Check sheet for the modelled part. Datum: model origin and axes. Units: mm. Coordinates: 2 decimals unless noted, no trailing zeros. Write each loop counter-clockwise with the first axis right and the second up, starting at its lowest first coordinate (ties: lowest second). Pieces come first, ordered by that corner, then holes. Notation, with made-up numbers: (-7, 56.5) - (49, 56.5) arc R23 cw to (49, 81.5) - close; hole circle Ø11 at (69.25, 73.5). An arc over 180 degrees is marked (long way). Use one line per item in the form item = value. Start each with the question number.
1. Scan lines: line 1 along X through (y, z) = (2.45, -15.5); line 2 along Z through (x, y) = (0, 0.75); line 3 along X through (y, z) = (1.8, -12). Record each from-to range of solid material in increasing order.
2. Cross-section at A-A on z = 0. Record the boundary of the cut face in (x, y), then the cut area to 3 significant figures.
3. Cross-section at B-B on x = 0. Record the boundary of the cut face in (y, z), then the cut area to 3 significant figures.
4. Go/stop test with a flat-tipped pin: pin 1 Ø10 at (x, z) = (-37.5, -12) entering from +Y. Record where the tip stops, or that it passes through.
5. Cross-section at C-C on y = 1.7. Give the number of separate pieces and of enclosed holes in the cut face, then the cut area to 3 significant figures.
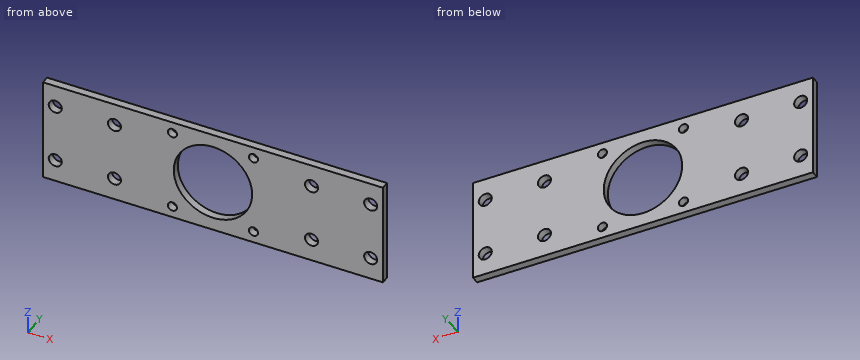
```python
from build123d import *

# Parameters (mm, degrees)
SKETCH1_W                  = 130
SKETCH1_H                  = 40
BOSS_EXTRUDE1_DEPTH        = 3
SKETCH2_R                  = 15
CUT_EXTRUDE1_DEPTH         = 69.0734897
F_5_0_5_DIAMETER_HOLE1_D   = 5
F_3_5_3_5_DIAMETER_HOLE1_D = 3.5


with BuildPart() as part:
    # Sketch1 → Boss-Extrude1 (new body)
    with BuildSketch(Plane(origin=(0, 0, 0), x_dir=(1, 0, 0), z_dir=(0, 1, 0))):
        Rectangle(SKETCH1_W, SKETCH1_H)
    extrude(amount=BOSS_EXTRUDE1_DEPTH)

    # Sketch2 → Cut-Extrude1 (cut, through all)
    with BuildSketch(Plane(origin=(0, 0, 0), x_dir=(1, 0, 0), z_dir=(0, 1, 0))):
        with Locations(Location((0, 0, 0), (0, 0, 270))):
            Circle(SKETCH2_R)
    extrude(amount=CUT_EXTRUDE1_DEPTH, mode=Mode.SUBTRACT)

    # Ø5.0 (5) Diameter Hole1 (through all)
    with Locations(Plane(origin=(0, 0, 0), x_dir=(-1, 0, 0), z_dir=(0, -1, 0))):
        with Locations((60.313708499, 11.313708499), (60.313708499, -11.313708499), (37.686291501, -11.313708499), (37.686291501, 11.313708499)):
            f_5_0_5_diameter_hole1 = Hole(F_5_0_5_DIAMETER_HOLE1_D / 2)

    # Mirror1: Ø5.0 (5) Diameter Hole1 across plane
    add(f_5_0_5_diameter_hole1.mirror(Plane(origin=(0, 0, 0), x_dir=(0, 0, 1), z_dir=(1, 0, 0))), mode=Mode.SUBTRACT)

    # Ø3.5 (3.5) Diameter Hole1 (through all)
    with Locations(Plane(origin=(0, 0, 0), x_dir=(-1, 0, 0), z_dir=(0, -1, 0))):
        with Locations((0, 0), (-15.5, 15.5), (15.5, -15.5), (15.5, 15.5), (-15.5, -15.5)):
            Hole(F_3_5_3_5_DIAMETER_HOLE1_D / 2)


solid = part.part
```
Final values:
q1.line_1 = -65 to -17.25, -13.75 to 13.75, 17.25 to 65
q1.line_2 = -20 to -15, 15 to 20
q1.line_3 = -65 to -62.72, -57.91 to -40.09, -35.28 to -9, 9 to 35.28, 40.09 to 57.91, 62.72 to 65
q2.outline = (-65, 0) - (-15, 0) - (-15, 3) - (-65, 3) - close; (15, 0) - (65, 0) - (65, 3) - (15, 3) - close
q2.area = 300 mm²
q3.outline = (0, -20) - (3, -20) - (3, -15) - (0, -15) - close; (0, 15) - (3, 15) - (3, 20) - (0, 20) - close
q3.area = 30.0 mm²
q4.pin_1 = 3
q5.separate_pieces = 1
q5.enclosed_holes = 13
q5.area = 4,300 mm²
